For this review, take the finished solid that the model builds, in its own axes (mm). Coordinates: 2 decimals unless noted, no trailing zeros. Write each loop counter-clockwise with the first axis right and the second up, starting at its lowest first coordinate (ties: lowest second). Pieces come first, ordered by that corner, then holes.
```python
from build123d import *

# Parameters (mm, degrees)
CROQUIS2_R                 = 4.35
ESPESOR_DE_BASE_FIJA_DEPTH = 15
CUT_EXTRUDE1_START         = -6
SKETCH2_R                  = 12.5
CUT_EXTRUDE1_DEPTH         = 6
FILLET1_START              = 9
FILLET1_DEPTH              = 7


with BuildPart() as part:
    # Croquis2 → Espesor de base fija (new body)
    with BuildSketch(Plane(origin=(0, 0, 0), x_dir=(1, 0, 0), z_dir=(0, 1, 0))):
        with BuildLine():
            ThreePointArc((131.556719836, 83.154307611), (0, 118.5), (-131.556719836, 83.154307611))
            ThreePointArc((-131.556719836, 83.154307611), (-136.117431676, 78.58743582), (-137.792102743, 72.354307611))
            ThreePointArc((-137.792102743, 72.354307611), (-102.624010348, -59.25), (-6.235382907, -155.508615221))
            ThreePointArc((-6.235382907, -155.508615221), (0, -157.17487164), (6.235382907, -155.508615221))
            ThreePointArc((6.235382907, -155.508615221), (102.624010348, -59.25), (137.792102743, 72.354307611))
            ThreePointArc((137.792102743, 72.354307611), (136.117431676, 78.58743582), (131.556719836, 83.154307611))
        make_face()
        with Locations(Location((0, -144, 0), (0, 0, 270))):
            Circle(CROQUIS2_R, mode=Mode.SUBTRACT)
        with Locations(Location((-124.707658145, 72, 0), (0, 0, 270))):
            Circle(CROQUIS2_R, mode=Mode.SUBTRACT)
        with Locations(Location((124.707658145, 72, 0), (0, 0, 270))):
            Circle(CROQUIS2_R, mode=Mode.SUBTRACT)
    extrude(amount=ESPESOR_DE_BASE_FIJA_DEPTH)

    # Sketch2 → Cut-Extrude1 (cut)
    with BuildSketch(Plane(origin=(0, 15, 0), x_dir=(1, 0, 0), z_dir=(0, 1, 0)).offset(CUT_EXTRUDE1_START)):
        with Locations((-125.292114129, 72.33743582)):
            Circle(SKETCH2_R)
        with Locations((125.292114129, 72.33743582)):
            Circle(SKETCH2_R)
        with Locations((0, -144.67487164)):
            Circle(SKETCH2_R)
    extrude(amount=CUT_EXTRUDE1_DEPTH, mode=Mode.SUBTRACT)

    # Fillet1: read off the stored shape, not the designer's step
    # Fillet1 outline → Fillet1 (cut)
    with BuildSketch(Plane(origin=(0, 0, 0), x_dir=(1, 0, 0), z_dir=(0, 1, 0)).offset(FILLET1_START)):
        with BuildLine():
            ThreePointArc((-117.884129659, 82.405790506), (-119.902519436, 86.861880767), (-117.152410353, 90.907562135))
            ThreePointArc((-117.152410353, 90.907562135), (-124.41497538, 87.143167542), (-131.556719836, 83.154307611))
            ThreePointArc((-131.556719836, 83.154307611), (-124.608814624, 84.818745919), (-117.884129659, 82.405790506))
        make_face()
        with BuildLine():
            ThreePointArc((131.556719836, 83.154307611), (124.41497538, 87.143167542), (117.152410353, 90.907562136))
            ThreePointArc((117.152410353, 90.907562136), (119.902519436, 86.861880767), (117.884129659, 82.405790506))
            ThreePointArc((117.884129659, 82.405790506), (124.608814624, 84.818745919), (131.556719836, 83.154307611))
        make_face()
        with BuildLine():
            ThreePointArc((-137.304463382, 56.003182413), (-135.175855082, 60.407687426), (-130.307572826, 60.887755734))
            ThreePointArc((-130.307572826, 60.887755734), (-135.759595995, 65.505026041), (-137.792102743, 72.354307611))
            ThreePointArc((-137.792102743, 72.354307611), (-137.675684548, 64.174945519), (-137.304463382, 56.003182413))
        make_face()
        with BuildLine():
            ThreePointArc((137.792102743, 72.354307611), (135.759595995, 65.505026041), (130.307572826, 60.887755734))
            ThreePointArc((130.307572826, 60.887755734), (135.175855082, 60.407687426), (137.304463382, 56.003182413))
            ThreePointArc((137.304463382, 56.003182413), (137.675684548, 64.174945519), (137.792102743, 72.354307611))
        make_face()
        with BuildLine():
            ThreePointArc((-12.423443168, -143.29354624), (-15.273335646, -147.269568193), (-20.152053029, -146.910744548))
            ThreePointArc((-20.152053029, -146.910744548), (-13.260709167, -151.31811306), (-6.235382907, -155.508615221))
            ThreePointArc((-6.235382907, -155.508615221), (-11.15078137, -150.323771959), (-12.423443168, -143.29354624))
        make_face()
        with BuildLine():
            ThreePointArc((6.235382907, -155.508615221), (13.260709167, -151.31811306), (20.152053029, -146.910744548))
            ThreePointArc((20.152053029, -146.910744548), (15.273335646, -147.269568193), (12.423443168, -143.29354624))
            ThreePointArc((12.423443168, -143.29354624), (11.15078137, -150.323771959), (6.235382907, -155.508615221))
        make_face()
    extrude(amount=FILLET1_DEPTH, mode=Mode.SUBTRACT)


solid = part.part
```
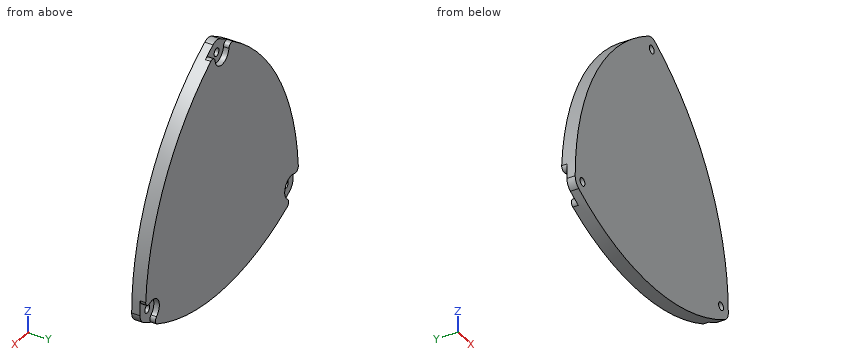
Q1. Clearance check with flat-ended pins moving along their axes: pin 1 Ø8 at (x, z) = (-124.71, -72) entering from +Y; pin 2 Ø12.5 at (x, z) = (6.5, 148) entering from +Y; pin 3 Ø3 at (x, y) = (-78, 2.5) entering from +Z; pin 4 Ø1.5 at (x, y) = (31.5, 4.5) entering from -Z. State where each tip first meets the part, or that it passes through.
Ans:
pin 1: passes through
pin 2: stops at y = 9
pin 3: stops at z = 96.59
pin 4: stops at z = -116.69
Q2. For probe 1 along X at (y, z) = (2.75, -72); probe 2 along Z at (x, y) = (0, 4.25); probe 3 along X at (y, z) = (3, -68), list the stretches that pass through material, from the lowest coordinate up.
Ans:
probe 1: x = -137.79 to -129.06, -120.36 to 120.36, 129.06 to 137.79
probe 2: z = -118.5 to 139.65, 148.35 to 157.17
probe 3: x = -137.76 to -126.42, -123 to 123, 126.42 to 137.76
Q3. Add section D-D (x = -41). State the section outline as (y, z) points, then the cut area to 3 significant figures.
Ans:
outline: (0, -115.28) - (15, -115.28) - (15, 131.59) - (0, 131.59) - close
area: 3,700 mm2
Q4. Add section C-C (z = 102.5). State the section outline as (x, y) points.
Ans:
outline: (-71.39, 0) - (71.39, 0) - (71.39, 15) - (-71.39, 15) - close
Q5. Add section B-B (y = 6). State the section outline as (x, z) points.
Ans:
outline: (-137.79, -72.35) arc R12.5 ccw to (-131.56, -83.15) arc R262.5 ccw to (131.56, -83.15) arc R12.5 ccw to (137.79, -72.35) arc R262.5 ccw to (6.24, 155.51) arc R12.5 ccw to (-6.24, 155.51) arc R262.5 ccw to start; hole circle Ø8.7 at (-124.71, -72); hole circle Ø8.7 at (0, 144); hole circle Ø8.7 at (124.71, -72)
Q6. Add section A-A (x = 0). State the section outline as (y, z) points.
Ans:
outline: (0, -118.5) - (15, -118.5) - (15, 132.17) - (9, 132.17) - (9, 139.65) - (0, 139.65) - close; (0, 148.35) - (9, 148.35) - (9, 157.17) - (0, 157.17) - close
